Answer from the drawing. Dimensions are ordinates in mm from the lowest x, y and z of the part. Coordinates: 2 decimals unless noted, no trailing zeros. Loops run counter-clockwise (first coordinate to the right, second up) from the corner with the lowest first, then second, coordinate; pieces in that order, holes last. Notation, with made-up numbers: M 70,73 L 97,73 A17 cw 97,101 Z; hole C 33,39 d2. An arc over 180 degrees is marked long. Answer as CSV lines item,"result". Start each with the question number.
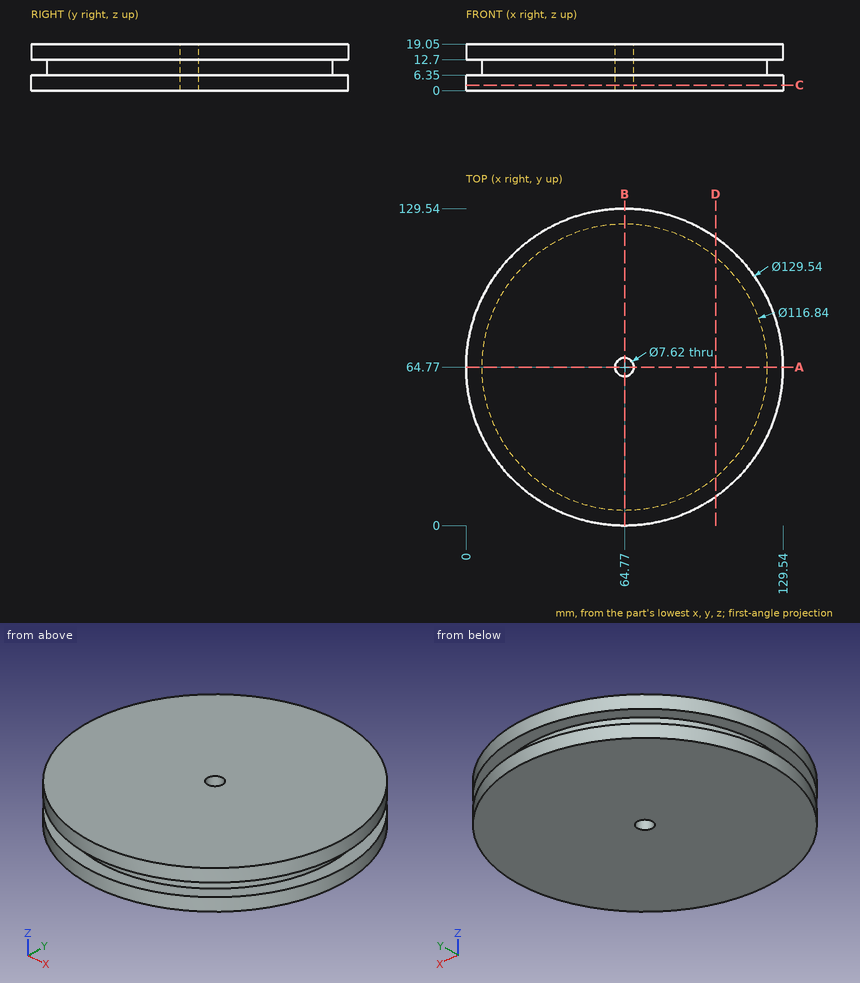
Item 1: Section A-A on y = 64.77 is taken. Determine the outline of the cut face in (x, z), then the cut area to 3 significant figures.
Item 2: Section D-D on x = 102 is taken. Determine the outline of the cut face in (y, z).
Item 3: Consider line 1 (X direction, y = 64.77, z = 5.5); line 2 (Z direction, x = 20, y = 18). Determine where each line is inside the solid, lowest interval first.
Item 4: Each of these flat-tipped pins is pushed along its axis until it touches: P1, Ø1.5, axis at y = 14.5, z = 15, coming from the -X side; P2, Ø6, axis at x = 60.5, z = 2, coming from the -Y side; P3, Ø8, axis at x = 70, z = 12.5, coming from the +Y side. Where does it stop, or does it pass through?
Item 5: Section C-C on z = 2.25 is taken. Determine the outline of the cut face in (x, y).
Results are:
1,outline,"M 0,0 L 60.96,0 L 60.96,19.05 L 0,19.05 L 0,12.7 L 6.35,12.7 L 6.35,6.35 L 0,6.35 Z; M 68.58,0 L 129.54,0 L 129.54,6.35 L 123.19,6.35 L 123.19,12.7 L 129.54,12.7 L 129.54,19.05 L 68.58,19.05 Z"
1,area,"2,240 mm²"
2,outline,"M 11.77,0 L 117.77,0 L 117.77,6.35 L 109.79,6.35 L 109.79,12.7 L 117.77,12.7 L 117.77,19.05 L 11.77,19.05 L 11.77,12.7 L 19.75,12.7 L 19.75,6.35 L 11.77,6.35 Z"
3,line 1,"0 to 60.96, 68.58 to 129.54"
3,line 2,"0 to 6.35, 12.7 to 19.05"
4,P1,"x = 23.02"
4,P2,"y = 0.01"
4,P3,"y = 129.53"
5,outline,"C 64.77,64.77 d129.54; hole C 64.77,64.77 d7.62"
